Source: CAD feature listing. Evaluate the final solid. Frame: model axes, mm. A direction names the side the tool comes from. Give positions to 0.01 mm unless a question says otherwise; leave off trailing zeros. Write each loop counter-clockwise with the first axis right and the second up, starting at its lowest first coordinate (ties: lowest second). Pieces come first, ordered by that corner, then holes. Notation, with made-up numbers: (88.5, 2.5) - (135.5, 2.5) arc R25 ccw to (135.5, 25.5) - close; hole circle Ø6 at (47, 46.25). An arc over 180 degrees is marked (long way). Answer as a JSON object with one key per item and string values. Group by question number.
from build123d import *
from OCP.BRepFilletAPI import BRepFilletAPI_MakeChamfer

# Parameters (mm, degrees)
BOSS_EXTRUDE1_DEPTH     = 25.4
CUT_EXTRUDE1_DEPTH      = 364.416353858
CUT_EXTRUDE1_DEPTH_BACK = 364.416353858
CUT_EXTRUDE2_DEPTH      = 243.106174261
CUT_EXTRUDE2_DEPTH_BACK = 243.106174261
SKETCH3_R               = 3.175
CHAMFER1_SIZE           = 12.7
CHAMFER1_SIZE2          = 15.677839289
CUT_EXTRUDE3_DEPTH      = 199.314331311
CUT_EXTRUDE3_DEPTH_BACK = 199.314331311
CUT_EXTRUDE4_DEPTH      = 209.332111666
CUT_EXTRUDE4_DEPTH_BACK = 209.332111666
SKETCH5_R               = 3.3655


with BuildPart() as part:
    # Sketch1 → Boss-Extrude1 (new body)
    with BuildSketch(Plane.XY):
        Polygon((32.258, 0), (-32.258, 0), (-32.258, -25.4), (-38.608, -25.4), (-38.608, 0), (-64.008, 0), (-171.45, 19.05), (-171.45, 117.668501525), (-152.4, 117.668501525), (-152.4, 41.468501525), (-38.608, 21.292615), (38.608, 21.292615), (152.4, 41.468501525), (152.4, 117.668501525), (171.45, 117.668501525), (171.45, 19.05), (64.008, 0), (38.608, 0), (38.608, -25.4), (32.258, -25.4), align=None)
    extrude(amount=BOSS_EXTRUDE1_DEPTH)

    # Sketch2 → Cut-Extrude1 (cut, two sides: drawn at the far end of the back side and taken through both)
    with BuildSketch(Plane(origin=(171.45, 0, 0), x_dir=(0, 0, -1), z_dir=(1, 0, 0)).offset(-CUT_EXTRUDE1_DEPTH_BACK)):
        with BuildLine():
            Line((-15.875, 117.668501525), (-9.525, 117.668501525))
            Line((-9.525, 117.668501525), (-9.525, 111.318501525))
            ThreePointArc((-9.525, 111.318501525), (-12.7, 108.143501525), (-15.875, 111.318501525))
            Line((-15.875, 111.318501525), (-15.875, 117.668501525))
        make_face()
    extrude(amount=CUT_EXTRUDE1_DEPTH + CUT_EXTRUDE1_DEPTH_BACK, mode=Mode.SUBTRACT)

    # Sketch3 → Cut-Extrude2 (cut, two sides: drawn at the far end of the back side and taken through both)
    with BuildSketch(Plane(origin=(38.608, 0, 0), x_dir=(0, 0, -1), z_dir=(1, 0, 0)).offset(-CUT_EXTRUDE2_DEPTH_BACK)):
        with Locations((-12.7, -12.7)):
            Circle(SKETCH3_R)
    extrude(amount=CUT_EXTRUDE2_DEPTH + CUT_EXTRUDE2_DEPTH_BACK, mode=Mode.SUBTRACT)

    # Chamfer1: one chamfer whose edges measure the first distance from different faces: ONE call of the kernel's chamfer builder (chamfer() names one face for all edges)
    chamfer1_edges_1 = [part.edges().sort_by_distance(p)[0] for p in [
        (-171.45, 19.05, 12.7),
    ]]
    chamfer1_side_1 = [part.faces().sort_by_distance(p)[0] for p in [
        (-171.45, 67.330500984, 12.7),
    ]]
    chamfer1_edges_2 = [part.edges().sort_by_distance(p)[0] for p in [
        (171.45, 19.05, 12.7),
    ]]
    chamfer1_side_2 = [part.faces().sort_by_distance(p)[0] for p in [
        (117.729, 9.525, 12.7),
    ]]
    chamfer1 = BRepFilletAPI_MakeChamfer(part.part.solid().wrapped)
    for e in chamfer1_edges_1:
        chamfer1.Add(CHAMFER1_SIZE, CHAMFER1_SIZE2, e.wrapped, chamfer1_side_1[0].wrapped)  # the first distance lies on this face
    for e in chamfer1_edges_2:
        chamfer1.Add(CHAMFER1_SIZE, CHAMFER1_SIZE2, e.wrapped, chamfer1_side_2[0].wrapped)  # the first distance lies on this face
    add(Compound.cast(chamfer1.Shape()), mode=Mode.REPLACE)

    # Sketch4 → Cut-Extrude3 (cut, two sides: drawn at the far end of the back side and taken through both)
    with BuildSketch(Plane(origin=(0, 21.292615, 0), x_dir=(1, 0, 0), z_dir=(0, 1, 0)).offset(-CUT_EXTRUDE3_DEPTH_BACK)):
        Polygon((15.875, 0), (15.875, -12.7), (-15.875, -12.7), (-15.875, -25.4), (141.747764855, -83.64087264), (246.478777591, -63.978728487), (187.893613379, 40.752284248), align=None)
    extrude(amount=CUT_EXTRUDE3_DEPTH + CUT_EXTRUDE3_DEPTH_BACK, mode=Mode.SUBTRACT)

    # Sketch5 → Cut-Extrude4 (cut, two sides: drawn at the far end of the back side and taken through both)
    with BuildSketch(Plane.XY.offset(12.7).offset(-CUT_EXTRUDE4_DEPTH_BACK)):
        with Locations((0, 10.6463075)):
            Circle(SKETCH5_R)
    extrude(amount=CUT_EXTRUDE4_DEPTH + CUT_EXTRUDE4_DEPTH_BACK, mode=Mode.SUBTRACT)


solid = part.part
Q1. First-contact query: pin 1 Ø7 at (x, y) = (-161.5, 115) entering from -Z; pin 2 Ø6.5 at (y, z) = (5.5, 16.5) entering from +X (3 decimals); pin 3 Ø12 at (y, z) = (-11, 4.5) entering from -X; pin 4 Ø12.5 at (x, z) = (-19, 10) entering from -Y. Flat tips, straight axial feed; report the tip coordinate or a pass-through.
Q2. Draft query along Y for faces 4 (the cylindrical face through (-35.5, -15.5, 11.2)), 5 (the flat face through (-18, 21.293, 10)), 6 (the flat face through (-35, -25.4, 13)). Return one class per face: released by +Y, released by -Y, zero draft, split by the parting line, or undercut.
Q3. Ray query, probe 1 along Z at (x, y) = (-36, -12.7) (3 decimals); probe 2 along Y at (x, z) = (-34, 12.7) (3 decimals); probe 3 along Y at (x, z) = (-15, 5.75). Return the intervals inside material, ascending. Write a range as [from, to].
Q4. Reachability of faces 1 (the flat face through (-162, 114, 15.875)), 2 (the flat face through (-51, 0, 13)), 3 (the flat face through (-32.258, -15.3, 15.3)) from +Z, -Z, +X, -X, +Y, -Y: full face, straight path, thin tool, end or side. Return the list, or none.
Q5. Section B-B on x = 0. Return the cut outline in (y, z).
Q6. Section A-A on y = -12.7. Return the cut outline in (x, z) (3 decimals).
Taken from the geometry:
{
 "1": {"pin 1": "stops at z = 0", "pin 2": "stops at x = -15.875", "pin 3": "stops at x = -38.61", "pin 4": "stops at y = 0"},
 "2": {"face 4": "undercut", "face 5": "released by +Y", "face 6": "released by -Y"},
 "3": {"probe 1": "z = [0, 9.525], [15.875, 25.4]", "probe 2": "y = [-25.4, -15.875], [-9.525, 21.293]", "probe 3": "y = [0, 21.29]"},
 "4": {"face 1": "+X, -X, +Y", "face 2": "+Z, -Z, -X, -Y", "face 3": "+Z, -Z, +X, -Y"},
 "5": {"outline": "(0, 0) - (7.28, 0) - (7.28, 12.7) - (0, 12.7) - close; (14.01, 0) - (21.29, 0) - (21.29, 12.7) - (14.01, 12.7) - close"},
 "6": {"outline": "(-38.608, 0) - (-32.258, 0) - (-32.258, 9.525) - (-38.608, 9.525) - close; (-38.608, 15.875) - (-32.258, 15.875) - (-32.258, 25.4) - (-38.608, 25.4) - close"}
}
